Part model, mm, in its own coordinate system. Round coordinates to 2 decimals unless told otherwise and drop trailing zeros. Write each question's results on one line, items separated by ' | '. Start each with the question number.
(1) Cut at A-A, the plane z = 1.3. Give the number of separate pieces and of enclosed holes in the cut face, then the cut area to 3 significant figures.
(2) Drill centre lines: L1, parallel to Y at x = -79.5, z = 1.6; L2, parallel to X at y = 114.5, z = 2.25; L3, parallel to X at y = 97, z = 3.95. Where is each one in solid material? Low to high.
(3) Flat gauge pins, fed straight in: P1, Ø1.5, axis at x = 88.5, z = 2.5, coming from the +Y side; P2, Ø2.5, axis at x = 87.5, z = 2.5, coming from the -Y side; P3, Ø1.5, axis at x = 88, z = 2, coming from the +Y side. Where does each tip first touch, or does it go through?
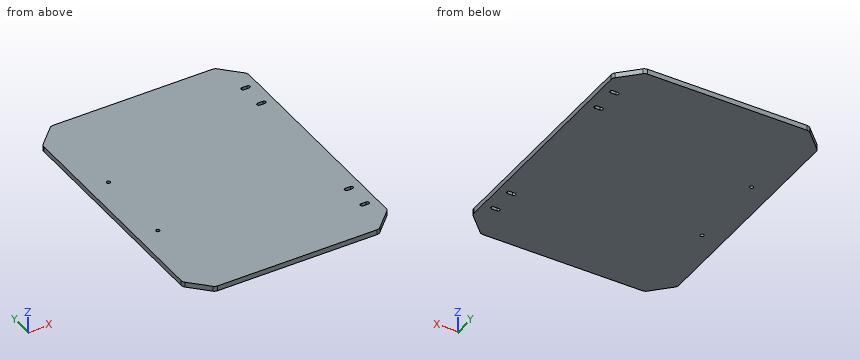
Autodesk Inventor part; units mm, degrees
ref_plane "YZ Plane" through (0, 0, 0) normal (1, 0, 0) x (0, 1, 0)
ref_plane "XZ Plane" through (0, 0, 0) normal (0, 1, 0) x (-1, 0, 0)
ref_plane "XY Plane" through (0, 0, 0) normal (0, 0, 1) x (1, 0, 0)
sketch "Hinges Screw Holes" plane through (0, 0, 0) normal (0, 0, 1) x (1, 0, 0)
  arc A0 (172, -72.429) -> (172, -68.929) centre (172, -70.679) ccw
  arc A1 (172, -97.929) -> (172, -94.429) centre (172, -96.179) ccw
  arc A2 (167, 97.929) -> (167, 94.429) centre (167, 96.179) ccw
  arc A3 (167, 72.429) -> (167, 68.929) centre (167, 70.679) ccw
  arc A4 (167, -68.929) -> (167, -72.429) centre (167, -70.679) ccw
  arc A5 (167, -94.429) -> (167, -97.929) centre (167, -96.179) ccw
  line L0 (167, 97.929) -> (172, 97.929)
  line L1 (167, 94.429) -> (172, 94.429)
  line L2 (167, 72.429) -> (172, 72.429)
  line L3 (167, 68.929) -> (172, 68.929)
  line L4 (167, -68.929) -> (172, -68.929)
  line L5 (167, -72.429) -> (172, -72.429)
  line L6 (167, -94.429) -> (172, -94.429)
  line L7 (167, -97.929) -> (172, -97.929)
  arc A6 (172, 94.429) -> (172, 97.929) centre (172, 96.179) ccw
  arc A7 (172, 68.929) -> (172, 72.429) centre (172, 70.679) ccw
  point P0 (169.5, 0)
  dimension "d28" = 3.5
  dimension "d29" = 3.5
  dimension "d30" = 25.5
  dimension "d31" = 3.5
  dimension "d32" = 3.5
  dimension "d33" = 25.5
  dimension "d34" = 141.358
  dimension "d35" = 3.5
  dimension "d36" = 3.5
  dimension "d37" = 25.5
  dimension "d38" = 3.5
  dimension "d39" = 3.5
  dimension "d40" = 25.5
  dimension "d41" = 141.358
  dimension "d42" = 5
sketch "Handle-Hole" plane through (0, 0, 0) normal (0, 0, 1) x (1, 0, 0)
  line L0 (-99.5, 50) -> (-69.5, 50)
  line L1 (-69.5, 50) -> (-69.5, -50)
  line L2 (-69.5, -50) -> (-99.5, -50)
  line L3 (-99.5, -50) -> (-99.5, 50)
  circle A0 centre (-87.5, 62) radius 1.75
  circle A1 centre (-57.5, 27.5) radius 1.75
  circle A2 centre (-57.5, -27.5) radius 1.75
  circle A3 centre (-87.5, -62) radius 1.75
  point P0 (-82.2826, 0)
  point P1 (-99.5, 0)
  point P2 (-99.5, 0)
  dimension "d11" = 30
  dimension "d12" = 100
  dimension "d13" = 3.5
  dimension "d14" = 3.5
  dimension "d15" = 3.5
  dimension "d16" = 3.5
  dimension "d17" = 55
  dimension "d19" = 12
  dimension "d20" = 12
  dimension "d22" = 12
sketch "Sketch1" plane through (0, 0, 0) normal (0, 0, 1) x (1, 0, 0)
  line L0 (-100, 133.5) -> (100, 133.5)
  line L1 (100, 133.5) -> (100, -133.5)
  line L2 (100, -133.5) -> (-100, -133.5)
  line L3 (-100, -133.5) -> (-100, 133.5)
  line L4 (99.5, 133) -> (-99.5, 133)
  line L5 (-99.5, 133) -> (-99.5, -133)
  line L6 (-99.5, -133) -> (99.5, -133)
  line L7 (99.5, -133) -> (99.5, 133)
  point P0 (0, 0)
  point P1 (0, 133.5)
  point P2 (-99.5, 0)
  dimension "d0" = 200
  dimension "d1" = 267
  dimension "d4" = 0.5
extrude "Extrusion1" add sketch "Sketch1" along normal blind 5 contours L7 L6 L5 L4
chamfer "Chamfer1" distance 20 angle 45 4 edges at (-99.5, -133, 2.5) (-99.5, 133, 2.5) (99.5, -133, 2.5) (99.5, 133, 2.5)
fillet "Fillet1" radius 5 8 edges at (-79.5, -133, 2.5) (79.5, -133, 2.5) (99.5, -113, 2.5) (99.5, 113, 2.5) (79.5, 133, 2.5) (-79.5, 133, 2.5) (-99.5, 113, 2.5) (-99.5, -113, 2.5)
sketch "Sketch2" plane through (0, 0, 5) normal (0, 0, 1) x (1, 0, 0)
  line L0 (99.5, -110.9289) -> (99.5, 110.9289)
  circle A0 centre (-79.5, 40) radius 1.75
  circle A1 centre (-79.5, -40) radius 1.75
  line L1 (-99.5, 110.9289) -> (-99.5, -110.9289)
  arc A2 (90, -72.429) -> (90, -68.929) centre (90, -70.679) ccw
  arc A3 (90, -97.929) -> (90, -94.429) centre (90, -96.179) ccw
  arc A4 (85, 97.929) -> (85, 94.429) centre (85, 96.179) ccw
  arc A5 (85, 72.429) -> (85, 68.929) centre (85, 70.679) ccw
  arc A6 (85, -68.929) -> (85, -72.429) centre (85, -70.679) ccw
  arc A7 (85, -94.429) -> (85, -97.929) centre (85, -96.179) ccw
  line L2 (85, 97.929) -> (90, 97.929)
  line L3 (85, 94.429) -> (90, 94.429)
  line L4 (85, 72.429) -> (90, 72.429)
  line L5 (85, 68.929) -> (90, 68.929)
  line L6 (85, -68.929) -> (90, -68.929)
  line L7 (85, -72.429) -> (90, -72.429)
  line L8 (85, -94.429) -> (90, -94.429)
  line L9 (85, -97.929) -> (90, -97.929)
  arc A8 (90, 94.429) -> (90, 97.929) centre (90, 96.179) ccw
  arc A9 (90, 68.929) -> (90, 72.429) centre (90, 70.679) ccw
  point P0 (0, 0)
  point P1 (0, 0)
  dimension "d43" = 141.358
  dimension "d44" = 70.679
  dimension "d45" = 9.5
  dimension "d46" = 9.5
  dimension "d47" = 3.5
  dimension "d48" = 80
  dimension "d49" = 20
  dimension "d50" = 40
extrude "Extrusion2" cut sketch "Sketch2" against normal blind 10
equation "\"d19\" = d20"
equation "\"d20\" = d21"
equation "\"d22\" = d21"
equation "\"d46\" = d45"
properties part number "Clear Right Side Door" material "Glass"
A:
1) separate pieces: 1 | enclosed holes: 6 | area: 52,000 mm2
2) L1: -132.55 to -41.75, -38.25 to 38.25, 41.75 to 132.55 | L2: -98 to 98 | L3: -99.5 to 83.45, 91.55 to 99.5
3) P1: y = 124.75 | P2: y = -126.25 | P3: y = 125.25
